For this review, take the finished solid that the model builds, in its own axes (mm). A direction names the side the tool comes from. Round coordinates to 2 decimals unless told otherwise and drop trailing zeros. Order: outer loops, then holes, each group sorted by start corner. A loop starts at its lowest first (then second) coordinate and runs counter-clockwise, first axis right, second up.
```python
from build123d import *

# Parameters (mm, degrees)
F0_W     = 25.4
F0_H     = 76.2
F1_DEPTH = 12.7
F2_DEPTH = 50.8
F3_DEPTH = 12.7
F5_DEPTH = 127.001
F6_W     = 76.2
F6_H     = 24.031783
F7_DEPTH = 76.201


with BuildPart() as f1:
    # F0 (on Top) → F1 (new body)
    with BuildSketch(Plane.XY):
        with Locations((-68.876286, -10.856101)):
            Rectangle(F0_W, F0_H)
    extrude(amount=F1_DEPTH)

    # F0 (on Top) → F2 (join)
    with BuildSketch(Plane.XY):
        Polygon((45.423714, 27.243899), (-56.176286, 27.243899), (-56.176286, -48.956101), (45.423714, -48.956101), (45.423714, -23.556101), (45.423714, 1.843899), align=None)
    extrude(amount=F2_DEPTH)

    # F0 (on Top) → F3 (join)
    with BuildSketch(Plane.XY):
        Polygon((70.823714, 27.243899), (45.423714, 27.243899), (45.423714, 1.843899), align=None)
        Polygon((45.423714, -23.556101), (45.423714, -48.956101), (70.823714, -48.956101), align=None)
    extrude(amount=F3_DEPTH)

    # F4 (on face) → F5 (cut, through all)
    with BuildSketch(Plane.YZ.offset(45.423714)):
        Polygon((-10.849641, 32.451563), (1.843899, 50.8), (-23.556101, 50.8), align=None)
    extrude(amount=-F5_DEPTH, mode=Mode.SUBTRACT)

    # F6 (on face) → F7 (cut, through all)
    with BuildSketch(Plane.XZ.offset(48.956101)):
        with Locations((-5.376286, 12.015891)):
            Rectangle(F6_W, F6_H)
    extrude(amount=-F7_DEPTH, mode=Mode.SUBTRACT)


solid = f1.part
```
Q1. Clearance check with flat-ended pins moving along their axes: pin 1 (12 mm diameter, centred on x = 13, y = -13, fed in from +Z); pin 2 (4 mm diameter, centred on y = -9, z = 34, fed in from +X); pin 3 (7 mm diameter, centred on y = -24.5, z = 7, fed in from +X). State where each tip first meets the part, or that it passes through.
Q2. Take a section at D-D, the plane y = -37. State the section outline as (x, z) points.
Q3. Mouldability with a two-part tool opening along Y and no side actions: class faces 5 (the face through (-6, -11, 24.032)), 6 (the face through (10, -48.956, 31)), 7 (the face through (-4.67, -17.29, 41.75)) as +Y half, -Y half, draft (parallel to the pull), parting line (faces both ways), or undercut.
Q4. Take a section at A-A, the plane z = 7. State the section outline as (x, y) points, plus the area to 3 significant figures.
Q5. Take a section at C-C, the plane z = 19. State the section outline as (x, y) points, plus the area to 3 significant figures.
Q6. Take a section at B-B, the plane x = -50.5. State the section outline as (y, z) points, plus the area to 3 significant figures.
Q7. Wall thickness on line 1 (X direction, y = -22, z = 16); line 2 (Z direction, x = -23.5, y = -38); line 3 (X direction, y = -38, z = 27): over which ranges is each line inside the solid? List them lowest first.
Q8. Tool access review of faces 1 (the face through (-56.176, -10, 31)), 2 (the face through (32.724, -11, 12)), 3 (the face through (58.3, -36.43, 6.26)), 4 (the face through (52, -42, 12.7)): name each direction out of +Z, -Z, +X, -X, +Y, -Y from which nothing blocks a thin tool from reaching the whole face with its end or side.
Working result:
1. pin 1: stops at z = 44.22
1. pin 2: stops at x = 45.42
1. pin 3: stops at x = 49.87
2. outline: (-81.58, 0) - (-43.48, 0) - (-43.48, 24.03) - (32.72, 24.03) - (32.72, 0) - (58.87, 0) - (58.87, 12.7) - (45.42, 12.7) - (45.42, 50.8) - (-56.18, 50.8) - (-56.18, 12.7) - (-81.58, 12.7) - close
3. face 5: draft
3. face 6: -Y half
3. face 7: undercut
4. outline: (-81.58, -48.96) - (-43.48, -48.96) - (-43.48, 27.24) - (-81.58, 27.24) - close; (32.72, -48.96) - (70.82, -48.96) - (45.42, -23.56) - (45.42, 1.84) - (70.82, 27.24) - (32.72, 27.24) - close
4. area: 4,520 mm2
5. outline: (-56.18, -48.96) - (-43.48, -48.96) - (-43.48, 27.24) - (-56.18, 27.24) - close; (32.72, -48.96) - (45.42, -48.96) - (45.42, 27.24) - (32.72, 27.24) - close
5. area: 1,940 mm2
6. outline: (-48.96, 0) - (27.24, 0) - (27.24, 50.8) - (1.84, 50.8) - (-10.85, 32.45) - (-23.56, 50.8) - (-48.96, 50.8) - close
6. area: 3,640 mm2
7. line 1: x = -56.18 to -43.48, 32.72 to 45.42
7. line 2: z = 24.03 to 50.8
7. line 3: x = -56.18 to 45.42
8. face 1: +Z, -X, +Y, -Y
8. face 2: -Z, +Y, -Y
8. face 3: +Z, -Z, +X
8. face 4: +Z, +X, +Y, -Y
